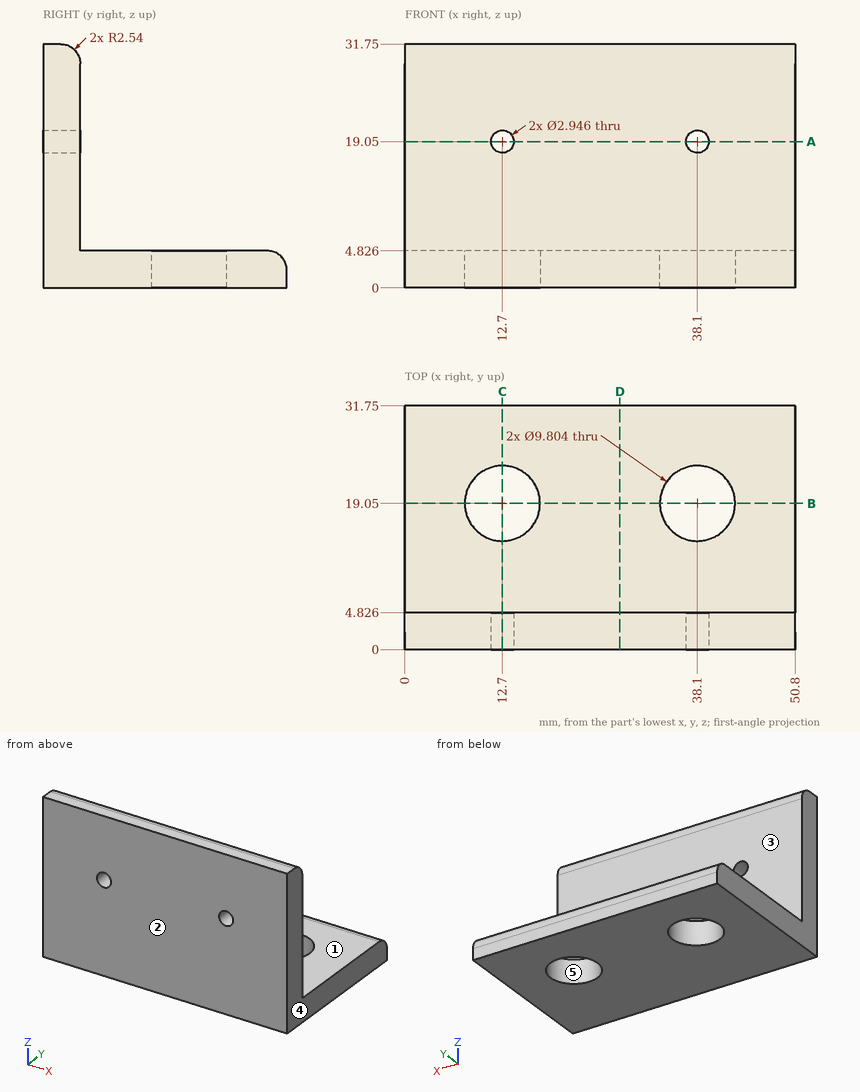
Job drawing, mm, ordinate dimensions from the low corner. One solid piece. A direction names the side the tool comes from. Give positions to 0.01 mm unless a question says otherwise; leave off trailing zeros. Loops run counter-clockwise (first coordinate to the right, second up) from the corner with the lowest first, then second, coordinate; pieces in that order, holes last. Notation, with made-up numbers: (29.25, 34.5) -> (53.25, 34.5) arc R29 ccw to (53.25, 69.5) -> close; hole circle Ø4 at (17, -1.5). An arc over 180 degrees is marked (long way). Use a Markdown table: item, result. Add a question column.
(1) Slice it at B-B on y = 19.05. List the corners of the cut face in (x, z).
(2) Slice it at D-D on x = 28. List the corners of the cut face in (y, z).
(3) Drop flat-ended pins along their axis: pin 1 Ø12 at (x, z) = (20.5, 16) entering from +Y; pin 2 Ø12 at (x, y) = (20.5, 22.5) entering from +Z; pin 3 Ø2 at (y, z) = (6.5, 13) entering from +X. Give the stop position or say it passes through.
(4) Tool access for the marked faces 1 and 2: list every direction of +Z, -Z, +X, -X, +Y, -Y with a clear straight run to the whole face (end or side of a thin tool).
(5) Wall check: line 1 along X through (y, z) = (2.65, 19.05); line 2 along Y through (x, z) = (38.1, 1.9); line 3 along Y through (x, z) = (44, 9.5). Give the ranges that are in metal, low to high.
(6) Slice it at C-C on x = 12.7. List the corners of the cut face in (y, z), and give its area (3 significant figures).
(7) Slice it at A-A on z = 19.05. List the corners of the cut face in (x, y).
(8) Mould opens along X. For the marked faces 3, 4 and 5 say: +X half, -X half, draft (parallel to the pull), parting line (faces both ways), or undercut.
Filled sheet:
| question | item | result |
|---|---|---|
| 1 | outline | (0, 0) -> (7.8, 0) -> (7.8, 4.83) -> (0, 4.83) -> close; (17.6, 0) -> (33.2, 0) -> (33.2, 4.83) -> (17.6, 4.83) -> close; (43, 0) -> (50.8, 0) -> (50.8, 4.83) -> (43, 4.83) -> close |
| 2 | outline | (0, 0) -> (31.75, 0) -> (31.75, 2.29) arc R2.54 ccw to (29.21, 4.83) -> (4.83, 4.83) -> (4.83, 29.21) arc R2.54 ccw to (2.29, 31.75) -> (0, 31.75) -> close |
| 3 | pin 1 | y = 4.83 |
| 3 | pin 2 | z = 4.83 |
| 3 | pin 3 | through |
| 4 | face 1 | +Z, +X, -X, +Y |
| 4 | face 2 | +Z, -Z, +X, -X, -Y |
| 5 | line 1 | 0 to 11.23, 14.17 to 36.63, 39.57 to 50.8 |
| 5 | line 2 | 0 to 14.15, 23.95 to 31.75 |
| 5 | line 3 | 0 to 4.83 |
| 6 | outline | (0, 0) -> (14.15, 0) -> (14.15, 4.83) -> (4.83, 4.83) -> (4.83, 17.58) -> (0, 17.58) -> close; (0, 20.52) -> (4.83, 20.52) -> (4.83, 29.21) arc R2.54 ccw to (2.29, 31.75) -> (0, 31.75) -> close; (23.95, 0) -> (31.75, 0) -> (31.75, 2.29) arc R2.54 ccw to (29.21, 4.83) -> (23.95, 4.83) -> close |
| 6 | area | 219 mm2 |
| 7 | outline | (0, 0) -> (11.23, 0) -> (11.23, 4.83) -> (0, 4.83) -> close; (14.17, 0) -> (36.63, 0) -> (36.63, 4.83) -> (14.17, 4.83) -> close; (39.57, 0) -> (50.8, 0) -> (50.8, 4.83) -> (39.57, 4.83) -> close |
| 8 | face 3 | draft |
| 8 | face 4 | +X half |
| 8 | face 5 | undercut |
